```python
from build123d import *

# Parameters (mm, degrees)
F0_W          = 107.3818355799
F0_H          = 89.936055243
F1_DEPTH      = 25.4
F2_R          = 18.0288778137
F3_DEPTH      = 25.4
F5_DEPTH      = 44.9690276215
F5_DEPTH_BACK = 25.4


with BuildPart() as f1:
    # F0 (on Top) → F1 (new body)
    with BuildSketch(Plane.XY):
        Rectangle(F0_W, F0_H)
    extrude(amount=F1_DEPTH)

    # F2 (on face) → F3 (join)
    with BuildSketch(Plane.XY.offset(25.4)):
        Circle(F2_R)
    extrude(amount=F3_DEPTH)

    # F4 (on Front) → F5 (cut, two sides)
    with BuildSketch(Plane.XZ) as f5_sk:
        Polygon((18.27981323, 50.8), (-18.6916068196, 50.8), (18.27981323, 37.2017361224), align=None)
    extrude(amount=-F5_DEPTH, mode=Mode.SUBTRACT)
    extrude(f5_sk.sketch, amount=F5_DEPTH_BACK, mode=Mode.SUBTRACT)


solid = f1.part
```
CAD build for the part. Positions are in the model's coordinates, mm. A direction names the side the tool comes from. Round coordinates to 2 decimals unless told otherwise and drop trailing zeros. Order: outer loops, then holes, each group sorted by start corner. A loop starts at its lowest first (then second) coordinate and runs counter-clockwise, first axis right, second up.
Q1. Which spindle directions (+Z, -Z, +X, -X, +Y, -Y) get a long thin tool onto all of the face, cutting with end or side? Do faces 1 (the flat face through (-1, 44.968, 13)), 2 (the flat face through (-1, -19, 25.4)). Say none if no direction does.
Q2. Wall check: L1, parallel to Z at x = 32.5, y = -15; L2, parallel to X at y = 3, z = 31; L3, parallel to Z at x = -12, y = -3.5. Give the ranges that are in metal, low to high.
Q3. Slice it at A-A (y = 4). Write the cut outline in (x, z).
Q4. Slice it at D-D (y = -26). Write the cut outline in (x, z).
Q5. Slice it at B-B (x = 0). Write the cut outline in (y, z), and give its area (3 significant figures).
Q6. Slice it at C-C (z = 29). Write the cut outline in (x, y).
Q7. Drop flat-ended pins along their axis: pin 1 (5 mm diameter, centred on y = 12.5, z = 45, fed in from -X); pin 2 (8 mm diameter, centred on x = 16, z = 31, fed in from +Y); pin 3 (12 mm diameter, centred on y = -11, z = 35.5, fed in from +X). Give the stop position or say it passes through.
Results below:
1. face 1: +Z, -Z, +X, -X, +Y
1. face 2: +Z
2. L1: z = 0 to 25.4
2. L2: x = -17.78 to 17.78
2. L3: z = 0 to 48.34
3. outline: (-53.69, 0) - (53.69, 0) - (53.69, 25.4) - (17.58, 25.4) - (17.58, 37.46) - (-17.58, 50.39) - (-17.58, 25.4) - (-53.69, 25.4) - close
4. outline: (-53.69, 0) - (53.69, 0) - (53.69, 25.4) - (-53.69, 25.4) - close
5. outline: (-44.97, 0) - (44.97, 0) - (44.97, 25.4) - (18.03, 25.4) - (18.03, 43.93) - (-18.03, 43.93) - (-18.03, 25.4) - (-44.97, 25.4) - close
5. area: 2,950 mm2
6. outline: circle Ø36.06 at (0, 0)
7. pin 1: stops at x = -15
7. pin 2: stops at y = 13.46
7. pin 3: stops at x = 17.32
